```python
from build123d import *

# Parameters (mm, degrees)
SKETCH_1_W          = 10
SKETCH_1_H          = 10
SKETCH_1_W_2        = 8
SKETCH_1_H_2        = 8
EXTRUDE_1_DEPTH     = 208
SKETCH_2_R          = 1.6
CUT_EXTRUDE_1_DEPTH = 209.300264042
SKETCH_3_R          = 1.6
CUT_EXTRUDE_2_DEPTH = 209.300264042
SKETCH_4_R          = 1.6
CUT_EXTRUDE_3_DEPTH = 209.300264042
SKETCH_5_R          = 1.6
CUT_EXTRUDE_4_DEPTH = 209.300264042


with BuildPart() as part:
    # ｽｹｯﾁ1 → ﾎﾞｽ - 押し出し1 (new body)
    with BuildSketch(Plane.XY):
        Rectangle(SKETCH_1_W, SKETCH_1_H)
        Rectangle(SKETCH_1_W_2, SKETCH_1_H_2, mode=Mode.SUBTRACT)
    extrude(amount=EXTRUDE_1_DEPTH)

    # ｽｹｯﾁ2 → ｶｯﾄ - 押し出し1 (cut, through all)
    with BuildSketch(Plane(origin=(5, 0, 0), x_dir=(0, 0, -1), z_dir=(1, 0, 0))):
        with Locations(Location((-203, 0, 0), (0, 0, 90))):
            Circle(SKETCH_2_R)
        with Locations(Location((-111.5, 0, 0), (0, 0, 90))):
            Circle(SKETCH_2_R)
        with Locations(Location((-96.5, 0, 0), (0, 0, 90))):
            Circle(SKETCH_2_R)
        with Locations(Location((-5, 0, 0), (0, 0, 90))):
            Circle(SKETCH_2_R)
    extrude(amount=-CUT_EXTRUDE_1_DEPTH, mode=Mode.SUBTRACT)

    # ｽｹｯﾁ3 → ｶｯﾄ - 押し出し2 (cut, through all)
    with BuildSketch(Plane(origin=(0, 5, 0), x_dir=(1, 0, 0), z_dir=(0, 1, 0))):
        with Locations(Location((0, -193, 0), (0, 0, 270))):
            Circle(SKETCH_3_R)
        with Locations(Location((0, -15, 0), (0, 0, 270))):
            Circle(SKETCH_3_R)
    extrude(amount=-CUT_EXTRUDE_2_DEPTH, mode=Mode.SUBTRACT)

    # ｽｹｯﾁ4 → ｶｯﾄ - 押し出し3 (cut, through all)
    with BuildSketch(Plane(origin=(5, 0, 0), x_dir=(0, 0, -1), z_dir=(1, 0, 0))):
        with Locations(Location((-129, 0, 0), (0, 0, 90))):
            Circle(SKETCH_4_R)
        with Locations(Location((-79, 0, 0), (0, 0, 90))):
            Circle(SKETCH_4_R)
    extrude(amount=-CUT_EXTRUDE_3_DEPTH, mode=Mode.SUBTRACT)

    # ｽｹｯﾁ5 → ｶｯﾄ - 押し出し4 (cut, through all)
    with BuildSketch(Plane(origin=(0, 5, 0), x_dir=(1, 0, 0), z_dir=(0, 1, 0))):
        with Locations(Location((0, -139, 0), (0, 0, 270))):
            Circle(SKETCH_5_R)
        with Locations(Location((0, -69, 0), (0, 0, 270))):
            Circle(SKETCH_5_R)
    extrude(amount=-CUT_EXTRUDE_4_DEPTH, mode=Mode.SUBTRACT)


solid = part.part
```
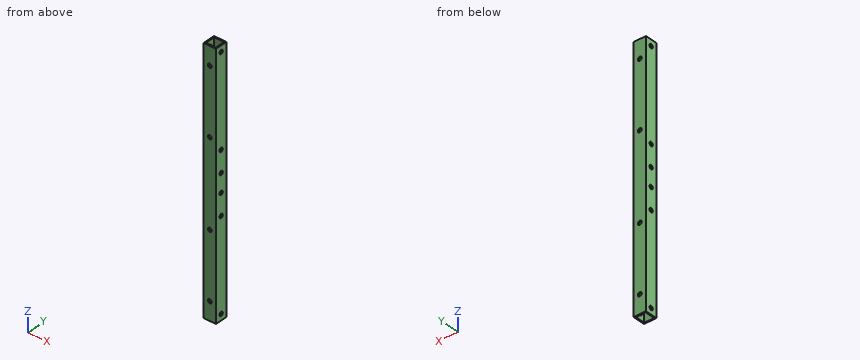
Source: CAD feature listing. Evaluate the final solid. Frame: model axes, mm. Coordinates: 2 decimals unless noted, no trailing zeros. Answer as a JSON object with one key per item and string values.
1. Contact query for flat-ended pins moving along their axis: P1, Ø4, axis at y = 0, z = 129, coming from the -X side; P2, Ø1.9, axis at x = 0, z = 69, coming from the -Y side. Output: stop coordinate, or through.
Evaluation:
{"P1": "x = -5", "P2": "through"}
2. Ray query, L1, parallel to Y at x = -3.25, z = 40.5; L2, parallel to Y at x = -4.75, z = 203. Return the intervals inside material, ascending.
Evaluation:
{"L1": "-5 to -4, 4 to 5", "L2": "-5 to -1.6, 1.6 to 5"}
3. Cut plane A-A on x = 0. State how many separate pieces and enclosed holes the cut face has, plus the area to 3 significant figures.
Evaluation:
{"separate pieces": "10", "enclosed holes": "0", "area": "390 mm^2"}
